Read the model definition and answer for the solid it produces. Units are mm, in the model's axes. A direction names the side the tool comes from. Coordinates: 2 decimals unless noted, no trailing zeros. Write each loop counter-clockwise with the first axis right and the second up, starting at its lowest first coordinate (ties: lowest second). Pieces come first, ordered by that corner, then holes. Notation, with made-up numbers: (50.25, -8.75) -> (92.25, -8.75) arc R20 ccw to (92.25, 4.25) -> close; hole circle Ø2 at (85, 69). An arc over 180 degrees is marked (long way). One line per item, written item: value. Start each with the question number.
from build123d import *

# Parameters (mm, degrees)
F0_W     = 50
F0_H     = 100
F1_DEPTH = 1850
F2_W     = 50.8
F2_H     = 101.6
F3_DEPTH = 50
F4_W     = 25
F4_H     = 100
F5_DEPTH = 50.8


# Not quite as in the source:
# - a feature names something its author has since deleted; it is built from what else it names


with BuildPart() as f1:
    # F0 (on Top) → F1 (new body)
    with BuildSketch(Plane.XY):
        Rectangle(F0_W, F0_H)
    extrude(amount=F1_DEPTH)

    # F2 (on Right) → F3 (cut, symmetric)
    with BuildSketch(Plane.YZ):
        with Locations((24.6, 1449.2)):
            Rectangle(F2_W, F2_H)
    extrude(amount=F3_DEPTH, both=True, mode=Mode.SUBTRACT)

    # F4 (on face) → F5 (cut)
    with BuildSketch(Plane.XY.offset(1850)):
        with Locations((-12.5, 0)):
            Rectangle(F4_W, F4_H)
    extrude(amount=-F5_DEPTH, mode=Mode.SUBTRACT)


solid = f1.part
1. For a pull along Z with two mould halves and no side action, classify faces 4 (the face through (0, 1, 0)), 5 (the face through (0, 24, 1500)), 6 (the face through (0, -50, 912)) as +Z half, -Z half, draft (parallel to the pull), parting line (faces both ways), or undercut.
2. A tool of negligible diameter and unlimited length cuts with its end or side. For faces 1 (the face through (0, 50, 1673)), 2 (the face through (0, -1, 1825)), 3 (the face through (0, 24, 1398.4)), from which of +Z, -Z, +X, -X, +Y, -Y can it reach the whole face along a straight path? Write none if from no direction.
3. Find the intervals of material crossed by probe 1 along Z at (x, y) = (21, 38); probe 2 along Z at (x, y) = (-21, 22); probe 3 along Z at (x, y) = (-7, -13), in increasing order. Write a range as from..to.
4. A cutting plane is placed at A-A on y = 28. Give the vertices of the cut face in (x, z).
5. A cutting plane is placed at B-B on x = 16.5. Give the vertices of the cut face in (y, z), then the cut area to 3 significant figures.
Derived:
1. face 4: -Z half
1. face 5: undercut
1. face 6: draft
2. face 1: +Z, -Z, +X, -X, +Y
2. face 2: +Z, -X, +Y, -Y
2. face 3: +X, -X, +Y
3. probe 1: z = 0..1398.4, 1500..1850
3. probe 2: z = 0..1398.4, 1500..1799.2
3. probe 3: z = 0..1799.2
4. outline: (-25, 0) -> (25, 0) -> (25, 1398.4) -> (-25, 1398.4) -> close; (-25, 1500) -> (25, 1500) -> (25, 1850) -> (0, 1850) -> (0, 1799.2) -> (-25, 1799.2) -> close
5. outline: (-50, 0) -> (50, 0) -> (50, 1398.4) -> (-0.8, 1398.4) -> (-0.8, 1500) -> (50, 1500) -> (50, 1850) -> (-50, 1850) -> close
5. area: 180,000 mm2
